```python
from build123d import *

# Parameters (mm, degrees)
SKETCH3_W          = 4.079746654
SKETCH3_H          = 4
CUT_EXTRUDE1_DEPTH = 51
CUT_EXTRUDE2_START = 11
CUT_EXTRUDE2_DEPTH = 1.7


with BuildPart() as part:
    # Sketch2 → Revolve1 (revolve)
    with BuildSketch(Plane(origin=(0, 0, 0), x_dir=(1, 0, 0), z_dir=(0, 1, 0)), mode=Mode.PRIVATE) as revolve1_sk:
        Polygon((0, 0), (-9.25, 0), (-9.25, 72), (-9.5, 72), (-9.5, 87), (-13, 87), (-13, 109), (-11, 109), (-11, 153), (-9.5, 153), (-9.5, 168), (0, 168), align=None)
    revolve(revolve1_sk.sketch.rotate(Axis((0, 0, 0), (0, 0, -1)), 180), axis=Axis((0, 0, 0), (0, 0, -1)))

    # Sketch3 → Cut-Extrude1 (cut)
    with BuildSketch(Plane.XY):
        with Locations((9.589873327, 0)):
            Rectangle(SKETCH3_W, SKETCH3_H)
    extrude(amount=-CUT_EXTRUDE1_DEPTH, mode=Mode.SUBTRACT)

    # Sketch4 → Cut-Extrude2 (cut)
    with BuildSketch(Plane(origin=(0, 0, 0), x_dir=(0, 0, -1), z_dir=(1, 0, 0)).offset(CUT_EXTRUDE2_START)):
        with BuildLine():
            Line((117, 2), (131, 2))
            ThreePointArc((131, 2), (133, 0), (131, -2))
            Line((131, -2), (117, -2))
            ThreePointArc((117, -2), (115, 0), (117, 2))
        make_face()
    extrude(amount=-CUT_EXTRUDE2_DEPTH, mode=Mode.SUBTRACT)


solid = part.part
```
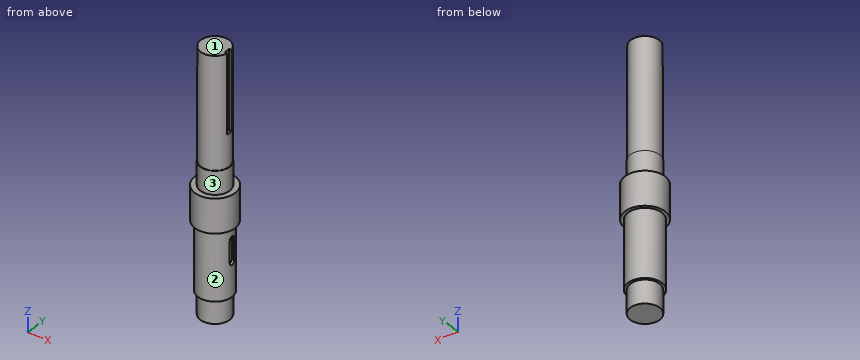
Input: part model. Units: mm. Frame: model coordinates. Face numbers are marked on the shaded views. A direction names the side the tool comes from. Round coordinates to 2 decimals unless told otherwise and drop trailing zeros. Loops run counter-clockwise (first coordinate to the right, second up) from the corner with the lowest first, then second, coordinate; pieces in that order, holes last. Notation, with made-up numbers: M 8,36 L 46,36 A20 ccw 46,46 Z; hole C -22.75,-7 d7. An arc over 180 degrees is marked long. Answer in a Markdown table with one row per item. Add a question column.
1. Ray query, probe 1 along X at (y, z) = (0.25, -68.5); probe 2 along Y at (x, z) = (-9.25, -98); probe 3 along Y at (x, z) = (-3.75, -42.5). Return the intervals inside material, ascending.
2. Section C-C (z = -157.5). Output: boundary loops of the cut face in (x, y).
3. Contact query for flat-ended pins moving along their axis: pin 1 (1 mm diameter, centred on x = -7.5, z = -47, fed in from -Y); pin 2 (0.8 mm diameter, centred on x = 10, z = -125.5, fed in from -Y); pin 3 (0.7 mm diameter, centred on x = 8.5, z = -36.5, fed in from +Y). Output: stop coordinate, or through.
4. Section D-D (z = -68.5). Output: boundary loops of the cut face in (x, y).
5. Set-up query: the marked faces 1, 2 and 3. Return all of +Z, -Z, +X, -X, +Y, -Y with unobstructed straight access to the full face (end or side cutting, diameter ignored); none if empty.
6. Section A-A (y = 0). Output: boundary loops of the cut face in (x, z).
7. Section B-B (x = 0). Output: boundary loops of the cut face in (y, z), and give its area (3 significant figures).
Values follow:
| question | item | result |
|---|---|---|
| 1 | probe 1 | -9.25 to 9.25 |
| 1 | probe 2 | -9.13 to 9.13 |
| 1 | probe 3 | -8.46 to 8.46 |
| 2 | outline | C 0,0 d19 |
| 3 | pin 1 | y = -6.05 |
| 3 | pin 2 | y = -5.37 |
| 3 | pin 3 | y = 4.37 |
| 4 | outline | C 0,0 d18.5 |
| 5 | face 1 | +Z, +X, -X, +Y, -Y |
| 5 | face 2 | -Z |
| 5 | face 3 | +Z |
| 6 | outline | M -13,-109 L -11,-109 L -11,-153 L -9.5,-153 L -9.5,-168 L 9.5,-168 L 9.5,-153 L 11,-153 L 11,-133 L 9.3,-133 L 9.3,-115 L 11,-115 L 11,-109 L 13,-109 L 13,-87 L 9.5,-87 L 9.5,-72 L 9.25,-72 L 9.25,-51 L 7.55,-51 L 7.55,0 L -9.25,0 L -9.25,-72 L -9.5,-72 L -9.5,-87 L -13,-87 Z |
| 7 | outline | M -13,-109 L -11,-109 L -11,-153 L -9.5,-153 L -9.5,-168 L 9.5,-168 L 9.5,-153 L 11,-153 L 11,-109 L 13,-109 L 13,-87 L 9.5,-87 L 9.5,-72 L 9.25,-72 L 9.25,0 L -9.25,0 L -9.25,-72 L -9.5,-72 L -9.5,-87 L -13,-87 Z |
| 7 | area | 3,440 mm^2 |
